Verification items for the finished model (mm, model axes). Face numbers are marked on the shaded views. A direction names the side the tool comes from. Coordinates: 2 decimals unless noted, no trailing zeros. Loops run counter-clockwise (first coordinate to the right, second up) from the corner with the lowest first, then second, coordinate; pieces in that order, holes last. Notation, with made-up numbers: M 70.25,68.5 L 119.25,68.5 A11 cw 119.25,83.5 Z; hole C 65.5,36.25 d4. An arc over 180 degrees is marked long. Write item = value, one per line. Start each with the question number.
```python
from build123d import *

# Parameters (mm, degrees)
SKETCH1_R           = 12.1
BOSS_EXTRUDE1_DEPTH = 52
SKETCH2_R           = 3.5
BOSS_EXTRUDE2_DEPTH = 2
BOSS_EXTRUDE3_DEPTH = 10


with BuildPart() as part:
    # Sketch1 → Boss-Extrude1 (new body)
    with BuildSketch(Plane.XY):
        Circle(SKETCH1_R)
    extrude(amount=BOSS_EXTRUDE1_DEPTH)

    # Sketch2 → Boss-Extrude2 (add)
    with BuildSketch(Plane.XY.offset(52)):
        Circle(SKETCH2_R)
    extrude(amount=BOSS_EXTRUDE2_DEPTH)

    # Sketch4 → Boss-Extrude3 (add)
    with BuildSketch(Plane.XY.offset(54)):
        with BuildLine():
            Line((-1.449347592, 1.378184152), (-1.449347592, -1.378184152))
            ThreePointArc((-1.449347592, -1.378184152), (2, 0), (-1.449347592, 1.378184152))
        make_face()
    extrude(amount=BOSS_EXTRUDE3_DEPTH)


solid = part.part
```
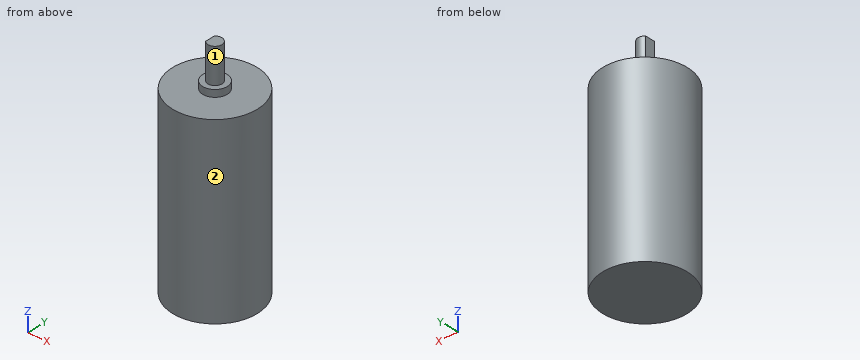
Q1. Sectioned sample at A-A on y = 0. Record the cut outline in (x, z), plus the area to 3 significant figures.
Q2. Scan lines: L1, parallel to Z at x = 1.25, y = 2.5; L2, parallel to Z at x = 4, y = 4; L3, parallel to X at y = 0.25, z = 20. Record each from-to range of solid material in increasing order. Write a range as [from, to].
Q3. Sectioned sample at C-C on z = 25.5. Record the cut outline in (x, y).
Q4. Gauge pin test, flat ends, axial feed: pin 1 (2 mm diameter, centred on x = -2, z = 56, fed in from +Y); pin 2 (1.5 mm diameter, centred on y = -4, z = 12.5, fed in from +X); pin 3 (12 mm diameter, centred on x = -7.5, y = -3.5, fed in from +Z); pin 4 (12 mm diameter, centred on x = -3.5, y = -5.5, fed in from +Z). Record the tip position at first contact, or that the pin passes through.
Q5. Sectioned sample at D-D on y = -2.75. Record the cut outline in (x, z), plus the area to 3 significant figures.
Q6. Sectioned sample at B-B on x = 0. Record the cut outline in (y, z).
Q7. Set-up check for the marked faces 1 and 2: record each of +Z, -Z, +X, -X, +Y, -Y from which the full face is reachable in a straight line by a thin tool's end or side.
Solutions:
q1.outline = M -12.1,0 L 12.1,0 L 12.1,52 L 3.5,52 L 3.5,54 L 2,54 L 2,64 L -1.45,64 L -1.45,54 L -3.5,54 L -3.5,52 L -12.1,52 Z
q1.area = 1,310 mm²
q2.L1 = [0, 54]
q2.L2 = [0, 52]
q2.L3 = [-12.1, 12.1]
q3.outline = C 0,0 d24.2
q4.pin_1 = 1.73
q4.pin_2 = 11.66
q4.pin_3 = 54
q4.pin_4 = 64
q5.outline = M -11.78,0 L 11.78,0 L 11.78,52 L 2.17,52 L 2.17,54 L -2.17,54 L -2.17,52 L -11.78,52 Z
q5.area = 1,230 mm²
q6.outline = M -12.1,0 L 12.1,0 L 12.1,52 L 3.5,52 L 3.5,54 L 2,54 L 2,64 L -2,64 L -2,54 L -3.5,54 L -3.5,52 L -12.1,52 Z
q7.face_1 = +Z
q7.face_2 = +Z, -Z
